from build123d import *

# Parameters (mm, degrees)
SKETCH1_R           = 2.5
BOSS_EXTRUDE1_DEPTH = 47.2
SKETCH2_R           = 3.5
BOSS_EXTRUDE2_DEPTH = 2
CHAMFER1_SIZE       = 1
SKETCH3_R           = 1.5
CUT_EXTRUDE1_DEPTH  = 5


with BuildPart() as part:
    # Sketch1 → Boss-Extrude1 (new body)
    with BuildSketch(Plane(origin=(0, 0, 0), x_dir=(1, 0, 0), z_dir=(0, 1, 0))):
        Circle(SKETCH1_R)
    extrude(amount=BOSS_EXTRUDE1_DEPTH)

    # Sketch2 → Boss-Extrude2 (add)
    with BuildSketch(Plane(origin=(0, 47.2, 0), x_dir=(1, 0, 0), z_dir=(0, 1, 0))):
        Circle(SKETCH2_R)
    extrude(amount=BOSS_EXTRUDE2_DEPTH)

    # Chamfer1
    chamfer1_edges = [part.edges().sort_by_distance(p)[0] for p in [
        (-3.5, 49.2, 0),
    ]]
    chamfer(chamfer1_edges, length=CHAMFER1_SIZE)

    # Sketch3 → Cut-Extrude1 (cut)
    with BuildSketch(Plane.XZ):
        Circle(SKETCH3_R)
    extrude(amount=-CUT_EXTRUDE1_DEPTH, mode=Mode.SUBTRACT)


solid = part.part
Design review of the part built by this model. Coordinates are the model's own, in mm. A direction names the side the tool comes from. Give positions to 0.01 mm unless a question says otherwise; leave off trailing zeros. Write each loop counter-clockwise with the first axis right and the second up, starting at its lowest first coordinate (ties: lowest second). Pieces come first, ordered by that corner, then holes. Notation, with made-up numbers: M -21.5,48 L 29.5,48 A20 ccw 29.5,84 Z; hole C 45.25,32 d3. An arc over 180 degrees is marked long. Return JSON: item names as keys, results as strings. Group by question number.
Item 1: Take a section at C-C (y = 3). Give the boundary of the cut face in (x, z).
Item 2: Take a section at A-A (z = 0). Give the boundary of the cut face in (x, y), plus the area to 3 significant figures.
Item 3: Take a section at B-B (x = 0). Give the boundary of the cut face in (y, z), plus the area to 3 significant figures.
Item 4: Take a section at D-D (y = 21). Give the boundary of the cut face in (x, z).
Item 5: Clearance check with flat-ended pins moving along their axes: pin 1 Ø1 at (x, y) = (2.5, 30.5) entering from +Z; pin 2 Ø3 at (x, y) = (2.5, 6.5) entering from -Z; pin 3 Ø1 at (y, z) = (26.5, -2) entering from -X. State where each tip first meets the part, or that it passes through.
Item 6: Tool access review of faces 1 (the cylindrical face through (-0.54, 23.27, 2.44)), 2 (the flat face through (0, 0, 2)): name each direction out of +Z, -Z, +X, -X, +Y, -Y from which nothing blocks a thin tool from reaching the whole face with its end or side.
Item 7: The part is to be moulded in two halves that separate along Z. For faces 3 (the flat face through (2, 47.2, 2)), 4 (the cylindrical face through (3.233, 47.693, 1.341)), 5 (the cylindrical face through (-1.5, 2.46, 0.07)), say which applies: pulls with the +Z half, pulls with the -Z half, needs draft (parallel to the pull), parting line crosses it, or undercut.
Item 8: Wall thickness on line 1 along Z through (x, y) = (0, 3.3); line 2 along X through (y, z) = (26, -2); line 3 along X through (y, z) = (32, 0): over which ranges is each line inside the solid? List them lowest first.
Return value:
{
 "1": {"outline": "C 0,0 d5; hole C 0,0 d3"},
 "2": {"outline": "M -3.5,47.2 L -2.5,47.2 L -2.5,0 L -1.5,0 L -1.5,5 L 1.5,5 L 1.5,0 L 2.5,0 L 2.5,47.2 L 3.5,47.2 L 3.5,48.2 L 2.5,49.2 L -2.5,49.2 L -3.5,48.2 Z", "area": "234 mm2"},
 "3": {"outline": "M 0,-2.5 L 47.2,-2.5 L 47.2,-3.5 L 48.2,-3.5 L 49.2,-2.5 L 49.2,2.5 L 48.2,3.5 L 47.2,3.5 L 47.2,2.5 L 0,2.5 L 0,1.5 L 5,1.5 L 5,-1.5 L 0,-1.5 Z", "area": "234 mm2"},
 "4": {"outline": "C 0,0 d5"},
 "5": {"pin 1": "stops at z = 1.5", "pin 2": "stops at z = -2.29", "pin 3": "stops at x = -2"},
 "6": {"face 1": "-Y", "face 2": "+Z, -Z, +X, -X, -Y"},
 "7": {"face 3": "needs draft", "face 4": "parting line crosses it", "face 5": "undercut"},
 "8": {"line 1": "z = -2.5 to -1.5, 1.5 to 2.5", "line 2": "x = -1.5 to 1.5", "line 3": "x = -2.5 to 2.5"}
}
